```python
from build123d import *

# Parameters (mm, degrees)
CROQUIS1_R              = 7.5
SALIENTE_EXTRUIR1_DEPTH = 26.15
REDONDEO1_R             = 1


with BuildPart() as part:
    # Croquis1 → Saliente-Extruir1 (new, symmetric)
    with BuildSketch(Plane.XY):
        Circle(CROQUIS1_R)
    extrude(amount=SALIENTE_EXTRUIR1_DEPTH, both=True)

    # Croquis2 → Taladro roscado M61 (revolve, cut)
    with BuildSketch(Plane(origin=(0, 0, 26.15), x_dir=(0, -1, 0), z_dir=(1, 0, 0))):
        Polygon((0, 0), (0, 18.502151548), (2.5, 17), (2.5, 0), align=None)
    taladro_roscado_m61 = revolve(axis=Axis((0, 0, 32.5), (0, 0, -1)), mode=Mode.SUBTRACT)

    # Redondeo1
    redondeo1_edges = [part.edges().sort_by_distance(p)[0] for p in [
        (-7.5, 0, -26.15),
        (-7.5, 0, 26.15),
    ]]
    fillet(redondeo1_edges, radius=REDONDEO1_R)

    # Simetría1: Taladro roscado M61 across plane
    add(taladro_roscado_m61.mirror(Plane.XY), mode=Mode.SUBTRACT)


solid = part.part
```
Could you check a few things on this model? Use its own coordinates, in mm. A direction names the side the tool comes from. Coordinates: 2 decimals unless noted, no trailing zeros. Loops run counter-clockwise (first coordinate to the right, second up) from the corner with the lowest first, then second, coordinate; pieces in that order, holes last. Notation, with made-up numbers: M 12.25,20 L 24.25,20 A12 ccw 24.25,43 Z; hole C -4.75,81.25 d8. An arc over 180 degrees is marked long. Put each result on its own line as item: value. Start each with the question number.
(1) Thinking about a two-plate mould opening in Y: for faces 3 (the face through (3, 0, -26.15)), 4 (the face through (-7.493, 0.33, 0.352)), 5 (the face through (2.44, 0.54, -17.77)), which applies, pulls with the +Y half, pulls with the -Y half, needs draft (parallel to the pull), parting line crosses it, or undercut?
(2) I need wall thicknesses on line 1 (Y direction, x = 0, z = -19.75); line 2 (Z direction, x = -2, y = -6.25); line 3 (X direction, y = 2.25, z = 17). Which ranges of each line are inside material? Lowest first, please. Write a range as from..to.
(3) For faces 1 (the face through (2.44, 0.54, 17.77)), 2 (the face through (3, 0, 26.15)), which set-ups out of +Z, -Z, +X, -X, +Y, -Y let a thin tool reach every point of the face, with its end or its side?
(4) Will these pins go through, and if not, where does the flat tip stop? P1, Ø4, axis at x = 0, y = 0, coming from the -Z side; P2, Ø2, axis at x = -1.5, z = -12, coming from the +Y side; P3, Ø2, axis at y = -5, z = 4.5, coming from the +X side.
(5) Suppose I cut it at A-A on z = 17.5. Please give me the cut outline in (x, y).
Solutions:
1. face 3: needs draft
1. face 4: parting line crosses it
1. face 5: undercut
2. line 1: y = -7.5..-2.5, 2.5..7.5
2. line 2: z = -26.15..26.15
2. line 3: x = -7.15..-1.09, 1.09..7.15
3. face 1: +Z
3. face 2: +Z, +X, -X, +Y, -Y
4. P1: stops at z = -8.85
4. P2: stops at y = 7.48
4. P3: stops at x = 6.34
5. outline: C 0,0 d15; hole C 0,0 d5
